Check sheet for the modelled part. Datum: model origin and axes. Units: mm. Face numbers are marked on the shaded views. A direction names the side the tool comes from. Coordinates: 2 decimals unless noted, no trailing zeros. Loops run counter-clockwise (first coordinate to the right, second up) from the corner with the lowest first, then second, coordinate; pieces in that order, holes last. Notation, with made-up numbers: M 88,-15 L 101,-15 A30 ccw 101,9 Z; hole C 60,89 d1. An arc over 180 degrees is marked long. Use CSV: the item, a comma, the result in double quotes. Start each with the question number.
(1) Section check C-C on z = -7.25. Record the cut outline in (x, y).
(2) Section check A-A on y = 10.25. Give the number of separate pieces and of enclosed holes in the cut face, and give its area (3 significant figures).
(3) Go/stop test with a flat-tipped pin: pin 1 Ø1.5 at (y, z) = (7, -6.5) entering from +X. Record where the tip stops, or that it passes through.
(4) Scan lines: line 1 (X direction, y = 10.75, z = -13); line 2 (Z direction, x = 13, y = 10.5); line 3 (Z direction, x = 12.25, y = 13.5). Record each from-to range of solid material in increasing order.
(5) Draft check along X on the marked faces 3, 4 and 5. Enter one of: pulls with the +X half, pulls with the -X half, needs draft (parallel to the pull), parting line crosses it, or undercut.
(6) Set-up check for the marked faces 1 and 2: record each of +Z, -Z, +X, -X, +Y, -Y from which the full face is reachable in a straight line by a thin tool's end or side.
from build123d import *

# Parameters (mm, degrees)
SKETCH1_W           = 14
SKETCH1_H           = 14
BOSS_EXTRUDE1_DEPTH = 2
SKETCH2_W           = 2.5
SKETCH2_H           = 1.5
BOSS_EXTRUDE2_DEPTH = 12
FILLET1_R           = 0.75


with BuildPart() as part:
    # Sketch1 → Boss-Extrude1 (new body)
    with BuildSketch(Plane(origin=(0, 0, 0), x_dir=(1, 0, 0), z_dir=(0, 1, 0))):
        with Locations((7, 7)):
            Rectangle(SKETCH1_W, SKETCH1_H)
    extrude(amount=BOSS_EXTRUDE1_DEPTH)

    # Sketch2 → Boss-Extrude2 (add)
    with BuildSketch(Plane(origin=(0, 2, 0), x_dir=(1, 0, 0), z_dir=(0, 1, 0))):
        with Locations((5.083333333, 0.75)):
            Rectangle(SKETCH2_W, SKETCH2_H)
        with Locations((1.25, 0.75)):
            Rectangle(SKETCH2_W, SKETCH2_H)
        with Locations((8.916666667, 0.75)):
            Rectangle(SKETCH2_W, SKETCH2_H)
        with Locations((12.75, 0.75)):
            Rectangle(SKETCH2_W, SKETCH2_H)
        with Locations((5.083333333, 4.916666667)):
            Rectangle(SKETCH2_W, SKETCH2_H)
        with Locations((8.916666667, 4.916666667)):
            Rectangle(SKETCH2_W, SKETCH2_H)
        with Locations((12.75, 4.916666667)):
            Rectangle(SKETCH2_W, SKETCH2_H)
        with Locations((5.083333333, 9.083333333)):
            Rectangle(SKETCH2_W, SKETCH2_H)
        with Locations((8.916666667, 9.083333333)):
            Rectangle(SKETCH2_W, SKETCH2_H)
        with Locations((12.75, 9.083333333)):
            Rectangle(SKETCH2_W, SKETCH2_H)
        with Locations((5.083333333, 13.25)):
            Rectangle(SKETCH2_W, SKETCH2_H)
        with Locations((8.916666667, 13.25)):
            Rectangle(SKETCH2_W, SKETCH2_H)
        with Locations((12.75, 13.25)):
            Rectangle(SKETCH2_W, SKETCH2_H)
        with Locations((1.25, 4.916666667)):
            Rectangle(SKETCH2_W, SKETCH2_H)
        with Locations((1.25, 9.083333333)):
            Rectangle(SKETCH2_W, SKETCH2_H)
        with Locations((1.25, 13.25)):
            Rectangle(SKETCH2_W, SKETCH2_H)
    extrude(amount=BOSS_EXTRUDE2_DEPTH)

    # Fillet1
    fillet1_edges = [part.edges().sort_by_distance(p)[0] for p in [
        (12.75, 14, -12.5),
        (8.916666667, 14, -12.5),
        (5.083333333, 14, -12.5),
        (1.25, 14, -12.5),
        (1.25, 14, -14),
        (5.083333333, 14, -14),
        (8.916666667, 14, -14),
        (12.75, 14, -14),
        (12.75, 14, -9.833333333),
        (8.916666667, 14, -9.833333333),
        (5.083333333, 14, -9.833333333),
        (1.25, 14, -9.833333333),
        (1.25, 14, -8.333333333),
        (5.083333333, 14, -8.333333333),
        (8.916666667, 14, -8.333333333),
        (12.75, 14, -8.333333333),
        (8.916666667, 14, -5.666666667),
        (12.75, 14, -5.666666667),
        (5.083333333, 14, -5.666666667),
        (1.25, 14, -5.666666667),
        (1.25, 14, -4.166666667),
        (5.083333333, 14, -4.166666667),
        (8.916666667, 14, -4.166666667),
        (12.75, 14, -4.166666667),
        (8.916666667, 14, 0),
        (12.75, 14, 0),
        (12.75, 14, -1.5),
        (8.916666667, 14, -1.5),
        (5.083333333, 14, -1.5),
        (5.083333333, 14, 0),
        (1.25, 14, -1.5),
        (1.25, 14, 0),
    ]]
    fillet(fillet1_edges, radius=FILLET1_R - 0.0001)  # a hair under: the kernel refuses the full size


solid = part.part
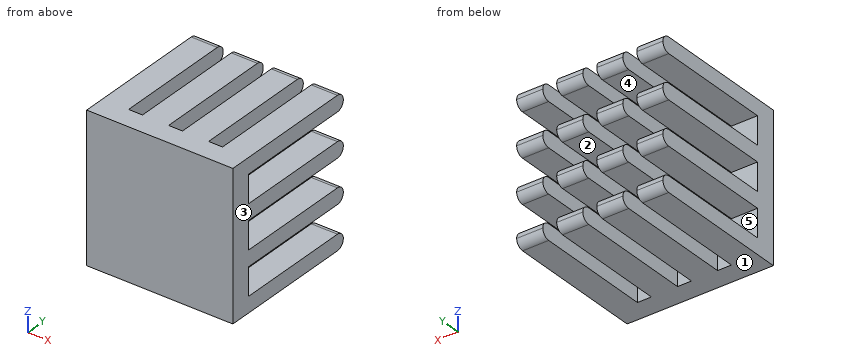
Outcome:
1,outline,"M 0,0 L 14,0 L 14,2 L 0,2 Z"
2,separate pieces,"16"
2,enclosed holes,"0"
2,area,"60.0 mm²"
3,pin 1,"passes through"
4,line 1,"x = 0 to 2.5, 3.83 to 6.33, 7.67 to 10.17, 11.5 to 14"
4,line 2,"z = -14 to -12.5, -9.83 to -8.33, -5.67 to -4.17, -1.5 to 0"
4,line 3,"z = -13.96 to -12.54, -9.79 to -8.38, -5.62 to -4.21, -1.46 to -0.04"
5,face 3,"pulls with the +X half"
5,face 4,"needs draft"
5,face 5,"undercut"
6,face 1,"-Z, +X, -X, +Y, -Y"
6,face 2,"+X, -X, +Y"
